For this review, take the finished solid that the model builds, in its own axes (mm). Give positions to 0.01 mm unless a question says otherwise; leave off trailing zeros. Order: outer loops, then holes, each group sorted by start corner. A loop starts at its lowest first (then second) coordinate and runs counter-clockwise, first axis right, second up. Notation, with made-up numbers: (14, 30) -> (57, 30) arc R15 ccw to (57, 49) -> close; hole circle Ø11 at (-22.75, -22). An arc over 180 degrees is marked (long way). One line per item, written item: value. Start each with the question number.
from build123d import *

# Parameters (mm, degrees)
SKETCH1_W           = 45
SKETCH1_H           = 29
SKETCH1_R           = 7.5
SKETCH1_R_2         = 2.5
BOSS_EXTRUDE1_DEPTH = 6


with BuildPart() as part:
    # Sketch1 → Boss-Extrude1 (new body)
    with BuildSketch(Plane.XY):
        with Locations((22.5, 14.5)):
            Rectangle(SKETCH1_W, SKETCH1_H)
        with Locations((22.5, 14.5)):
            Circle(SKETCH1_R, mode=Mode.SUBTRACT)
        with Locations((7.5, 14.5)):
            Circle(SKETCH1_R_2, mode=Mode.SUBTRACT)
        with Locations(Location((37.5, 14.5, 0), (0, 0, 180))):
            Circle(SKETCH1_R_2, mode=Mode.SUBTRACT)
    extrude(amount=BOSS_EXTRUDE1_DEPTH)


solid = part.part
Q1. For line 1 along Y through (x, z) = (7.5, 2.35); line 2 along X through (y, z) = (12.25, 3.5); line 3 along Y through (x, z) = (22.5, 3), list the stretches that pass through material, from the lowest coordinate up.
Q2. For pin 1 Ø3 at (x, y) = (7.5, 14.5) entering from +Z, flat-tipped, find the tip position at first contact; note if it passes through.
Q3. Take a section at B-B (x = 22.5). State the section outline as (y, z) points, and give its area (3 significant figures).
Q4. Take a section at D-D (y = 10.5). State the section outline as (x, z) points.
Q5. Take a section at C-C (z = 3.05). State the section outline as (x, y) points.
Q6. Take a section at A-A (y = 14.5). State the section outline as (x, z) points, and give its area (3 significant figures).
Q7. Mouldability with a two-part tool opening along X and no side actions: class faces 1 (the flat face through (0, 14, 3)), 2 (the flat face through (45, 14, 3)), 3 (the cylindrical face through (8.65, 12.28, 2.96)), 4 (the flat face through (22, 29, 3)) as pulls with the +X half, pulls with the -X half, needs draft (parallel to the pull), parting line crosses it, or undercut.
Answers below:
1. line 1: y = 0 to 12, 17 to 29
1. line 2: x = 0 to 6.41, 8.59 to 15.35, 29.65 to 36.41, 38.59 to 45
1. line 3: y = 0 to 7, 22 to 29
2. pin 1: passes through
3. outline: (0, 0) -> (7, 0) -> (7, 6) -> (0, 6) -> close; (22, 0) -> (29, 0) -> (29, 6) -> (22, 6) -> close
3. area: 84.0 mm²
4. outline: (0, 0) -> (16.16, 0) -> (16.16, 6) -> (0, 6) -> close; (28.84, 0) -> (45, 0) -> (45, 6) -> (28.84, 6) -> close
5. outline: (0, 0) -> (45, 0) -> (45, 29) -> (0, 29) -> close; hole circle Ø5 at (7.5, 14.5); hole circle Ø15 at (22.5, 14.5); hole circle Ø5 at (37.5, 14.5)
6. outline: (0, 0) -> (5, 0) -> (5, 6) -> (0, 6) -> close; (10, 0) -> (15, 0) -> (15, 6) -> (10, 6) -> close; (30, 0) -> (35, 0) -> (35, 6) -> (30, 6) -> close; (40, 0) -> (45, 0) -> (45, 6) -> (40, 6) -> close
6. area: 120 mm²
7. face 1: pulls with the -X half
7. face 2: pulls with the +X half
7. face 3: undercut
7. face 4: needs draft
